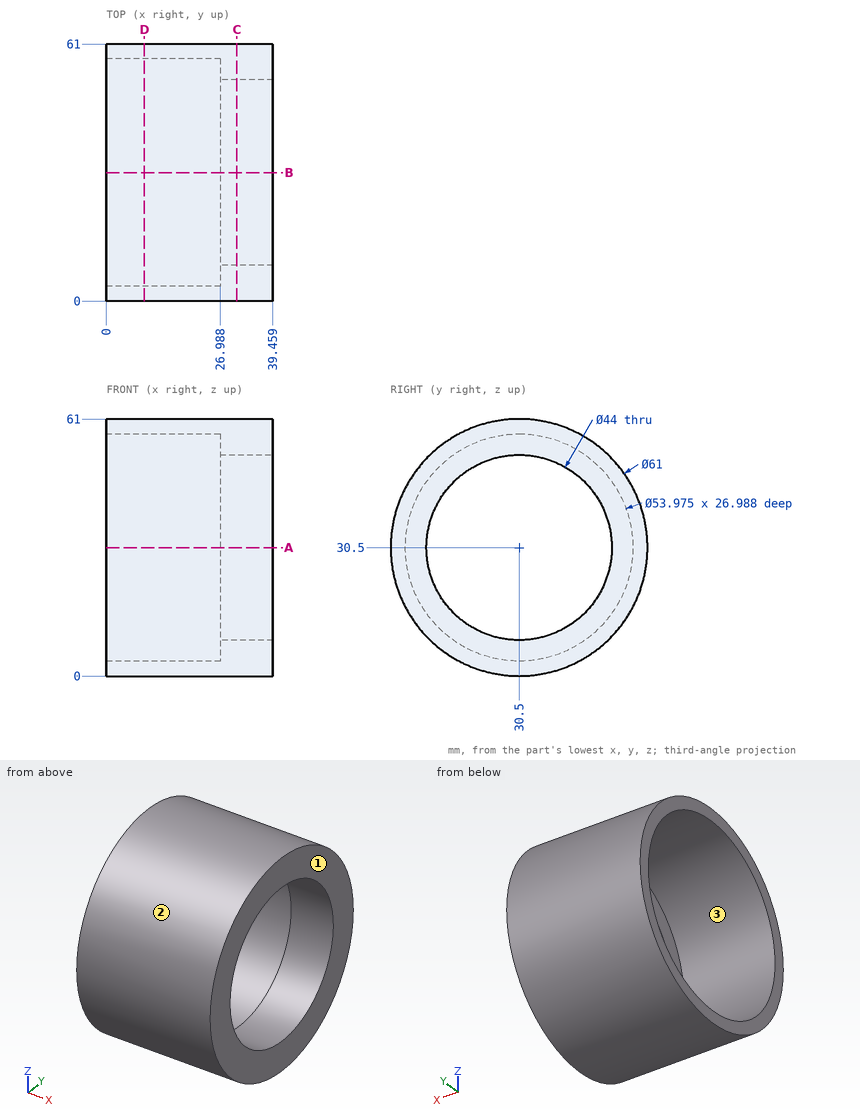
Answer from the drawing. Dimensions are ordinates in mm from the lowest x, y and z of the part. Coordinates: 2 decimals unless noted, no trailing zeros. Write each loop counter-clockwise with the first axis right and the second up, starting at its lowest first coordinate (ties: lowest second). Pieces come first, ordered by that corner, then holes. Notation, with made-up numbers: M -10.5,26 L 14.5,26 A27 cw 14.5,63 Z; hole C 12.5,-16 d3. An arc over 180 degrees is marked long. Use one line per item in the form item = value. Start each with the question number.
1. The part is cut by section C-C (x = 31). Give the vertices of the cut face in (y, z), plus the area to 3 significant figures.
2. Straight lines are drawn through the part: probe 1 along Z at (x, y) = (35, 30) (1 decimal); probe 2 along Y at (x, z) = (15, 30) (1 decimal). For each, find the intervals that lie inside material, in ascending order. Write a range as from..to.
3. Each of these flat-tipped pins is pushed along its axis until it touches: P1, Ø4, axis at x = 31.5, z = 48.5, coming from the -Y side (1 decimal); P2, Ø6, axis at x = 7, y = 14, coming from the -Z side; P3, Ø5, axis at x = 29, y = 21, coming from the -Z side (1 decimal). Where does it stop, or does it pass through?
4. The part is cut by section A-A (z = 30.5). Give the vertices of the cut face in (x, y).
5. The part is cut by section D-D (x = 9). Give the vertices of the cut face in (y, z) (1 decimal).
6. The mould has two halves that part along Z. Classify the marked faces 1, 2 and 3: released by +Z, released by -Z, zero draft, split by the parting line, or undercut.
Evaluation:
q1.outline = C 30.5,30.5 d61; hole C 30.5,30.5 d44
q1.area = 1,400 mm^2
q2.probe_1 = 0..8.5, 52.5..61
q2.probe_2 = 0..3.5, 57.5..61
q3.P1 = 4.5
q3.P2 = 3.15
q3.P3 = 0.8
q4.outline = M 0,0 L 39.46,0 L 39.46,8.5 L 26.99,8.5 L 26.99,3.51 L 0,3.51 Z; M 0,57.49 L 26.99,57.49 L 26.99,52.5 L 39.46,52.5 L 39.46,61 L 0,61 Z
q5.outline = C 30.5,30.5 d61; hole C 30.5,30.5 d54
q6.face_1 = zero draft
q6.face_2 = split by the parting line
q6.face_3 = undercut
